Work out the finished part from the listing and answer in its coordinate system (mm). A direction names the side the tool comes from. Round coordinates to 2 decimals unless told otherwise and drop trailing zeros. Loops run counter-clockwise (first coordinate to the right, second up) from the corner with the lowest first, then second, coordinate; pieces in that order, holes last. Notation, with made-up numbers: (73.5, -37) - (119.5, -37) arc R12 ccw to (119.5, -32) - close; hole circle Ø8 at (8.25, 4). An arc over 180 degrees is marked (long way). Answer as CSV lines item,"result". Start each with the question number.
Q1. Section B-B on y = 5.25 is taken. Count the separate pieces of the cut face and the enclosed holes in it, then the cut area to 3 significant figures.
Q2. Section A-A on z = 81 is taken. Write down the section's boundary in (x, y), then the cut area to 3 significant figures.
Q3. The mould has two halves that part along Y. Classify faces 4 (the face through (1, 6, 66)), 5 (the face through (4, 0, 8)), 6 (the face through (5, 6, 32)): +Y half, -Y half, draft (parallel to the pull), parting line (faces both ways), or undercut.
Q4. Straight lines are drawn through the part: L1, parallel to Z at x = 0.75, y = 7; L2, parallel to X at y = 5.5, z = 81; L3, parallel to Z at x = 5.75, y = 1.75. For each, find the intervals that lie inside material, in ascending order. Write a range as [from, to].
Q5. Each of these flat-tipped pins is pushed along its axis until it touches: pin 1 Ø4 at (x, z) = (5.25, 21) entering from +Y; pin 2 Ø2.5 at (x, z) = (5.5, 61) entering from -Y; pin 3 Ø2.5 at (y, z) = (5.5, 30) entering from -X. Where does it stop, or does it pass through?
Q6. For faces 1 (the face through (0, 4, 13)), 2 (the face through (5, 1, 86)), 3 (the face through (2.5, 3, 91)), determine the directions among +Z, -Z, +X, -X, +Y, -Y from which every point of the face is accessible in a straight line to the end or side of a thin tool.
```python
from build123d import *

# Parameters (mm, degrees)
SKETCH_W               = 8.5
SKETCH_H               = 8.5
PAD_DEPTH              = 113.5
SKETCH001_W            = 10
SKETCH001_H            = 10
POCKET_DEPTH           = 2.5
LINEARPATTERN_COUNT    = 4
LINEARPATTERN_PITCH    = 20
SKETCH002_W            = 10
SKETCH002_H            = 10
POCKET001_DEPTH        = 2.5
LINEARPATTERN001_COUNT = 4
LINEARPATTERN001_PITCH = 20
FILLET_R               = 1
SKETCH003_R            = 1.25
POCKET002_DEPTH        = 6.001
LINEARPATTERN002_COUNT = 4
LINEARPATTERN002_PITCH = 20
SKETCH004_R            = 1.25
POCKET003_DEPTH        = 6.001
LINEARPATTERN003_COUNT = 4
LINEARPATTERN003_PITCH = 20
SKETCH005_R            = 2.5
POCKET004_DEPTH        = 12


with BuildPart() as part:
    # Sketch → Pad (new body)
    with BuildSketch(Plane.XY):
        with Locations((4.25, 4.25)):
            Rectangle(SKETCH_W, SKETCH_H)
    extrude(amount=PAD_DEPTH)

    # Sketch001 → Pocket (cut)
    with BuildSketch(Plane.XZ):
        with Locations((4.410969, 21)):
            Rectangle(SKETCH001_W, SKETCH001_H)
    pocket = extrude(amount=-POCKET_DEPTH, mode=Mode.SUBTRACT)

    # LinearPattern: Pocket ×4
    with Locations(*[(0, 0, i * LINEARPATTERN_PITCH) for i in range(1, LINEARPATTERN_COUNT)]):
        add(pocket, mode=Mode.SUBTRACT)

    # Sketch002 → Pocket001 (cut)
    with BuildSketch(Plane(origin=(0, 0, 0), x_dir=(0, -1, 0), z_dir=(-1, 0, 0))):
        with Locations((-4.326825, 31)):
            Rectangle(SKETCH002_W, SKETCH002_H)
    pocket001 = extrude(amount=-POCKET001_DEPTH, mode=Mode.SUBTRACT)

    # LinearPattern001: Pocket001 ×4
    with Locations(*[(0, 0, i * LINEARPATTERN001_PITCH) for i in range(1, LINEARPATTERN001_COUNT)]):
        add(pocket001, mode=Mode.SUBTRACT)

    # Fillet
    fillet_edges = [part.edges().sort_by_distance(p)[0] for p in [
        (8.5, 8.5, 56.75),
    ]]
    fillet(fillet_edges, radius=FILLET_R)

    # Sketch003 → Pocket002 (cut, through all)
    with BuildSketch(Plane.XZ.offset(-2.5)):
        with Locations((5.25, 21)):
            Circle(SKETCH003_R)
    pocket002 = extrude(amount=-POCKET002_DEPTH, mode=Mode.SUBTRACT)

    # LinearPattern002: Pocket002 ×4
    with Locations(*[(0, 0, i * LINEARPATTERN002_PITCH) for i in range(1, LINEARPATTERN002_COUNT)]):
        add(pocket002, mode=Mode.SUBTRACT)

    # Sketch004 → Pocket003 (cut, through all)
    with BuildSketch(Plane(origin=(2.5, 0, 0), x_dir=(0, -1, 0), z_dir=(-1, 0, 0))):
        with Locations((-5.25, 31)):
            Circle(SKETCH004_R)
    pocket003 = extrude(amount=-POCKET003_DEPTH, mode=Mode.SUBTRACT)

    # LinearPattern003: Pocket003 ×4
    with Locations(*[(0, 0, i * LINEARPATTERN003_PITCH) for i in range(1, LINEARPATTERN003_COUNT)]):
        add(pocket003, mode=Mode.SUBTRACT)

    # Sketch005 → Pocket004 (cut)
    with BuildSketch(Plane.XY.offset(113.5)):
        with Locations((4.25, 4.25)):
            Circle(SKETCH005_R)
    extrude(amount=-POCKET004_DEPTH, mode=Mode.SUBTRACT)


solid = part.part
```
Findings:
1,separate pieces,"5"
1,enclosed holes,"4"
1,area,"730 mm^2"
2,outline,"(0, 2.5) - (4, 2.5) - (4, 8.5) - (0, 8.5) - close; (6.5, 2.5) - (8.5, 2.5) - (8.5, 7.5) arc R1 ccw to (7.5, 8.5) - (6.5, 8.5) - close"
2,area,"35.8 mm^2"
3,face 4,"draft"
3,face 5,"-Y half"
3,face 6,"undercut"
4,L1,"z = [0, 26], [36, 46], [56, 66], [76, 86], [96, 113.5]"
4,L2,"x = [0, 4], [6.5, 8.5]"
4,L3,"z = [0, 16], [26, 36], [46, 56], [66, 76], [86, 113.5]"
5,pin 1,"stops at y = 8.5"
5,pin 2,"stops at y = 2.5"
5,pin 3,"stops at x = 2.5"
6,face 1,"+Z, -Z, -X, +Y, -Y"
6,face 2,"+X, -X, -Y"
6,face 3,"-X, +Y, -Y"
